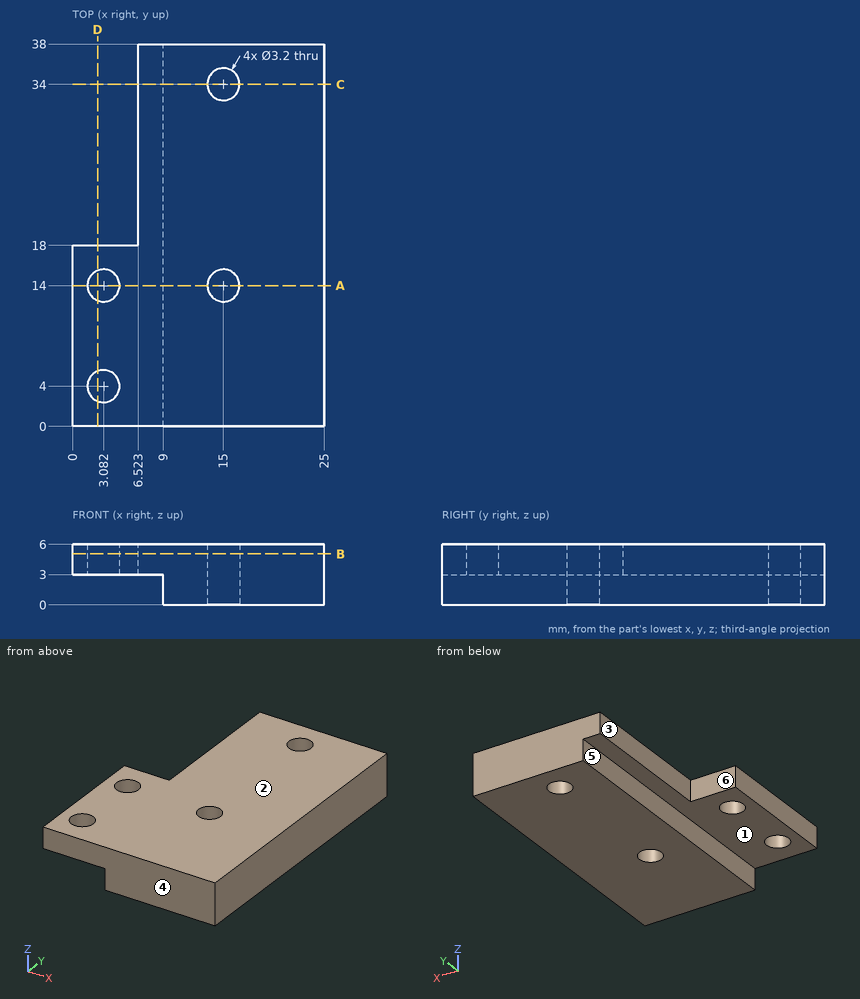
Can you work these out from the drawing? Everything is in mm from the part's minimum corner. A direction names the side the tool comes from. Coordinates: 2 decimals unless noted, no trailing zeros. Write each loop counter-clockwise with the first axis right and the second up, starting at its lowest first coordinate (ties: lowest second). Pieces come first, ordered by that corner, then holes. Notation, with made-up numbers: (-4.5, 0) -> (11.5, 0) arc R17 cw to (11.5, 10) -> close; hole circle Ø9 at (52, 8). An arc over 180 degrees is marked (long way). Return JSON: item names as keys, results as strings.
(1) Imagine slicing it at C-C, the plane y = 34. Please give me the cut outline in (x, z).
Numbers:
{"outline": "(6.52, 3) -> (9, 3) -> (9, 0) -> (13.4, 0) -> (13.4, 6) -> (6.52, 6) -> close; (16.6, 0) -> (25, 0) -> (25, 6) -> (16.6, 6) -> close"}
(2) I need wall thicknesses on L1, parallel to Y at x = 15, z = 2.35; L2, parallel to Y at x = 13.75, z = 5.45; L3, parallel to X at y = 4.5, z = 1.4. Which ranges of each line are inside material? Lowest first, please.
Numbers:
{"L1": "y = 0 to 12.4, 15.6 to 32.4, 35.6 to 38", "L2": "y = 0 to 13, 15 to 33, 35 to 38", "L3": "x = 9 to 25"}
(3) Imagine slicing it at D-D, the plane x = 2.5. Please give me the cut outline in (y, z), then the cut area to 3 significant figures.
Numbers:
{"outline": "(0, 3) -> (2.51, 3) -> (2.51, 6) -> (0, 6) -> close; (5.49, 3) -> (12.51, 3) -> (12.51, 6) -> (5.49, 6) -> close; (15.49, 3) -> (18, 3) -> (18, 6) -> (15.49, 6) -> close", "area": "36.1 mm2"}
(4) Which directions (+Z, -Z, +X, -X, +Y, -Y) give clear straight access to the entire face, cutting with the end or side of a thin tool? Please do the marked faces 4, 5 and 6.
Numbers:
{"face 4": "+Z, -Z, +X, -X, -Y", "face 5": "-Z, -X, +Y, -Y", "face 6": "+Z, -Z, -X, +Y"}
(5) I'm going to push flat-ended pins straight in: pin 1 (3 mm diameter, centred on y = 20.5, z = 3, fed in from -X); pin 2 (0.9 mm diameter, centred on x = 2.5, z = 4, fed in from +Y); pin 3 (2.5 mm diameter, centred on x = 3.08, y = 4, fed in from +Z); pin 4 (8 mm diameter, centred on x = 3, y = 28, fed in from -Z). Where does each tip first touch, or does it pass through?
Numbers:
{"pin 1": "stops at x = 6.52", "pin 2": "stops at y = 18", "pin 3": "passes through", "pin 4": "stops at z = 3"}
(6) We'd pull the mould along Z, two halves only. Please class the marked faces 1, 2 and 3: +Z half, -Z half, draft (parallel to the pull), parting line (faces both ways), or undercut.
Numbers:
{"face 1": "-Z half", "face 2": "+Z half", "face 3": "draft"}
(7) Imagine slicing it at B-B, the plane z = 5.05. Please give me the cut outline in (x, y).
Numbers:
{"outline": "(0, 0) -> (25, 0) -> (25, 38) -> (6.52, 38) -> (6.52, 18) -> (0, 18) -> close; hole circle Ø3.2 at (3.08, 4); hole circle Ø3.2 at (3.08, 14); hole circle Ø3.2 at (15, 14); hole circle Ø3.2 at (15, 34)"}
(8) Imagine slicing it at A-A, the plane y = 14. Please give me the cut outline in (x, z).
Numbers:
{"outline": "(0, 3) -> (1.48, 3) -> (1.48, 6) -> (0, 6) -> close; (4.68, 3) -> (9, 3) -> (9, 0) -> (13.4, 0) -> (13.4, 6) -> (4.68, 6) -> close; (16.6, 0) -> (25, 0) -> (25, 6) -> (16.6, 6) -> close"}
